Design review of the part built by this model. Coordinates are the model's own, in mm. A direction names the side the tool comes from. Coordinates: 2 decimals unless noted, no trailing zeros. Write each loop counter-clockwise with the first axis right and the second up, starting at its lowest first coordinate (ties: lowest second). Pieces come first, ordered by that corner, then holes. Notation, with made-up numbers: (44, -26) -> (89, -26) arc R15 ccw to (89, -18) -> close; hole circle Ø5 at (-33.5, 44.25). An arc over 180 degrees is marked (long way). One line per question, with ' | ' between items. Start each with the question number.
Q1. For P1, Ø5, axis at x = 28.5, z = 6.5, coming from the +Y side; P2, Ø8, axis at x = -2.5, z = 26, coming from the -Y side; P3, Ø5, axis at y = 1, z = 26.5, coming from the +X side; P4, Ø1.8, axis at x = 3, z = 5, coming from the -Y side, all flat-tipped, find the tip position at first contact; note any pin that passes through.
Q2. Add section A-A on z = 5. State the section outline as (x, y) points.
Q3. Add section C-C on x = 3. State the section outline as (y, z) points.
Q4. Add section B-B on y = 6. State the section outline as (x, z) points, and give its area (3 significant figures).
Q5. Add section D-D on x = 15.5. State the section outline as (y, z) points.
Q6. For faces 5 (the flat face through (18, 5, 40)), 6 (the flat face through (-5.303, 2.465, 24.721)), 7 (the flat face through (31, 2, 5)), 8 (the flat face through (-2, 3, 12)), list the 3-axis set-ups (+Z, -Z, +X, -X, +Y, -Y) from which the entire face can be reached by the end or side of a thin tool; tool diameter is ignored.
Q7. Draft analysis for pull direction Y (two halves, no side actions). For faces 1 (the flat face through (21.2, -0.29, 23.4)), 2 (the flat face through (18.827, 6.38, 27.126)), 3 (the flat face through (1.7, 5, 3.8)), 4 (the flat face through (1.7, 0, 3.8)), state which applies: pulls with the +Y half, pulls with the -Y half, needs draft (parallel to the pull), parting line crosses it, or undercut.
Q8. Wall thickness on probe 1 along X at (y, z) = (1.6, 5); probe 2 along Z at (x, y) = (16.5, 3.5); probe 3 along Y at (x, z) = (4, 2.5): over which ranges is each line inside the solid? List them lowest first.
from build123d import *

# Parameters (mm, degrees)
SKETCH1_R           = 1.5
BOSS_EXTRUDE1_DEPTH = 5
BOSS_EXTRUDE2_DEPTH = 2.5
BOSS_EXTRUDE3_DEPTH = 2.5
SKETCH6_R           = 7.6
CUT_EXTRUDE1_DEPTH  = 1.2
SKETCH8_R           = 6.6
CUT_EXTRUDE2_DEPTH  = 56.938163239
CUT_EXTRUDE5_START  = -9.689111
CUT_EXTRUDE5_DEPTH  = 9.689111
FILLET1_R           = 5
SKETCH9_R           = 4
CUT_EXTRUDE6_DEPTH  = 56.783708254


with BuildPart() as part:
    # Sketch1 → Boss-Extrude1 (new body)
    with BuildSketch(Plane(origin=(0, 0, 0), x_dir=(1, 0, 0), z_dir=(0, 1, 0))):
        Polygon((0, 0), (6, 0), (6, -10), (25, -10), (25, 0), (31, 0), (31, -10), (33, -10), (33, -24.378221735), (25.810889132, -36.830127019), (24.078838325, -35.830127019), (19.078838325, -44.490381057), (13.882685902, -41.490381057), (18.882685902, -32.830127019), (2.42820323, -23.330127019), (-2.57179677, -31.990381057), (-7.767949192, -28.990381057), (-2.767949192, -20.330127019), (-4.5, -19.330127019), (-2, -15), (-2, -10), (0, -10), align=None)
        with Locations(Location((3, -5, 0), (0, 0, 270))):
            Circle(SKETCH1_R, mode=Mode.SUBTRACT)
        with Locations(Location((28, -5, 0), (0, 0, 90))):
            Circle(SKETCH1_R, mode=Mode.SUBTRACT)
        with Locations(Location((-2.669872981, -26.160254038, 0), (0, 0, 270))):
            Circle(SKETCH1_R, mode=Mode.SUBTRACT)
        with Locations(Location((18.980762114, -38.660254038, 0), (0, 0, 270))):
            Circle(SKETCH1_R, mode=Mode.SUBTRACT)
    extrude(amount=BOSS_EXTRUDE1_DEPTH)

    # Sketch2 → Boss-Extrude2 (add)
    with BuildSketch(Plane(origin=(0, 5, 0), x_dir=(1, 0, 0), z_dir=(0, 1, 0))):
        Polygon((-2, -10), (33, -10), (33, -24.378221735), (25.810889132, -36.830127019), (-4.5, -19.330127019), (-2, -15), align=None)
    extrude(amount=BOSS_EXTRUDE2_DEPTH)

    # Sketch3 → Boss-Extrude3 (add)
    with BuildSketch(Plane.XZ):
        Polygon((-2, 10), (33, 10), (33, 24.378221735), (25.810889132, 36.830127019), (-4.5, 19.330127019), (-2, 15), align=None)
    extrude(amount=BOSS_EXTRUDE3_DEPTH)

    # Sketch6 → Cut-Extrude1 (cut)
    with BuildSketch(Plane(origin=(0, 4.09, 0), x_dir=(1, 0, 0), z_dir=(0, 1, 0))):
        with Locations(Location((15.5, -19.689110868, 0), (0, 0, 270))):
            Circle(SKETCH6_R)
    cut_extrude1 = extrude(amount=CUT_EXTRUDE1_DEPTH, mode=Mode.SUBTRACT)

    # Sketch8 → Cut-Extrude2 (cut, through all)
    with BuildSketch(Plane(origin=(0, 5.29, 0), x_dir=(1, 0, 0), z_dir=(0, 1, 0))):
        with Locations(Location((15.5, -19.689110868, 0), (0, 0, 270))):
            Circle(SKETCH8_R)
    cut_extrude2 = extrude(amount=CUT_EXTRUDE2_DEPTH, mode=Mode.SUBTRACT)

    # Sketch5 → Cut-Extrude5 (cut)
    with BuildSketch(Plane(origin=(-9.495190528, 0, 16.446152423), x_dir=(0.8660254037844386, 0, 0.5000000000000003), z_dir=(-0.5000000000000003, 0, 0.8660254037844386)).offset(CUT_EXTRUDE5_START)):
        Polygon((16.667949192, 7.5), (16.667949192, 5.29), (15.667949192, 5.29), (15.667949192, 4.09), (23.267949192, 4.09), (30.867949192, 4.09), (30.867949192, 5.29), (29.867949192, 5.29), (29.867949192, 7.5), align=None)
    cut_extrude5 = extrude(amount=CUT_EXTRUDE5_DEPTH, mode=Mode.SUBTRACT)

    # Mirror1: Cut-Extrude1, Cut-Extrude2, Cut-Extrude5 across plane
    add(cut_extrude1.mirror(Plane.ZX.offset(2.5)), mode=Mode.SUBTRACT)
    add(cut_extrude2.mirror(Plane.ZX.offset(2.5)), mode=Mode.SUBTRACT)
    add(cut_extrude5.mirror(Plane.ZX.offset(2.5)), mode=Mode.SUBTRACT)

    # Fillet1
    fillet1_edges = [part.edges().sort_by_distance(p)[0] for p in [
        (33, 2.5, 24.378221735),
        (-2, 2.5, 15),
    ]]
    fillet(fillet1_edges, radius=FILLET1_R)

    # Sketch9 → Cut-Extrude6 (cut, through all)
    with BuildSketch(Plane(origin=(0, 4.09, 0), x_dir=(1, 0, 0), z_dir=(0, 1, 0))):
        with Locations(Location((15.5, -19.689110868, 0), (0, 0, 270))):
            Circle(SKETCH9_R)
    extrude(amount=-CUT_EXTRUDE6_DEPTH, mode=Mode.SUBTRACT)


solid = part.part
Output values:
1) P1: stops at y = 5 | P2: stops at y = 0 | P3: stops at x = 32.91 | P4: passes through
2) outline: (0, 0) -> (1.5, 0) -> (1.5, 5) -> (0, 5) -> close; (4.5, 0) -> (6, 0) -> (6, 5) -> (4.5, 5) -> close; (25, 0) -> (26.5, 0) -> (26.5, 5) -> (25, 5) -> close; (29.5, 0) -> (31, 0) -> (31, 5) -> (29.5, 5) -> close
3) outline: (-2.5, 10) -> (0, 10) -> (0, 6.5) -> (5, 6.5) -> (5, 10) -> (7.5, 10) -> (7.5, 23.66) -> (-2.5, 23.66) -> close; (0, 0) -> (5, 0) -> (5, 3.5) -> (0, 3.5) -> close
4) outline: (-4.5, 19.33) -> (-2.67, 16.16) arc R5 cw to (-2, 13.66) -> (-2, 10) -> (33, 10) -> (33, 23.04) arc R5 ccw to (32.33, 25.54) -> (25.81, 36.83) -> (16.37, 31.38) -> (21.22, 22.99) arc R6.6 cw to (9.78, 16.39) -> (4.94, 24.78) -> close | area: 482 mm2
5) outline: (-2.5, 10) -> (7.5, 10) -> (7.5, 13.09) -> (5.29, 13.09) -> (5.29, 12.09) -> (4.09, 12.09) -> (4.09, 15.69) -> (0.91, 15.69) -> (0.91, 12.09) -> (-0.29, 12.09) -> (-0.29, 13.09) -> (-2.5, 13.09) -> close; (0, 38.69) -> (5, 38.69) -> (5, 42.42) -> (0, 42.42) -> close; (0.91, 23.69) -> (4.09, 23.69) -> (4.09, 30.88) -> (0.91, 30.88) -> close
6) face 5: +Z, -X, +Y | face 6: -X, +Y, -Y | face 7: -Z, +X, +Y, -Y | face 8: -Z, -X, +Y, -Y
7) face 1: undercut | face 2: needs draft | face 3: pulls with the +Y half | face 4: pulls with the -Y half
8) probe 1: x = 0 to 1.5, 4.5 to 6, 25 to 26.5, 29.5 to 31 | probe 2: z = 10 to 15.82, 23.56 to 31.45, 36.96 to 43 | probe 3: y = 0 to 5
